Input: part model. Units: mm. Frame: model coordinates. Coordinates: 2 decimals unless noted, no trailing zeros. Write each loop counter-clockwise with the first axis right and the second up, starting at its lowest first coordinate (ties: lowest second). Pieces come first, ordered by that corner, then holes. Notation, with made-up numbers: (-3, -32.75) - (48, -32.75) arc R8 cw to (48, -21.75) - close; hole circle Ø2 at (18, 12.5). An arc over 180 degrees is marked (long way). One line per question, with ' | ' between items. Start each with the question number.
1) Section query C-C on y = 54. Return loops of the section in (x, z), and give its area (3 significant figures).
2) Section query B-B on x = -64.5. Return loops of the section in (y, z), and give its area (3 significant figures).
3) First-contact query: P1, Ø4, axis at x = -110, y = 73, coming from the +Z side; P2, Ø1.5, axis at x = 68.5, y = -59.5, coming from the -Z side; P3, Ø3, axis at x = -113.5, z = 8, coming from the +Y side. Flat tips, straight axial feed; report the tip coordinate or a pass-through.
4) Section query A-A on y = -46.5. Return loops of the section in (x, z), and give its area (3 significant figures).
5) Line query: line 1 (Z direction, x = -8.5, y = 60.5); line 2 (Y direction, x = -72, z = 8.5); line 3 (Y direction, x = -104.5, z = 6). Output: solid intervals per line, ascending.
6) Draft query along X for faces 1 (the flat face through (-2, 1, 0)), 2 (the conical face through (-117.49, -20.18, 7.24)), 3 (the conical face through (123.848, -86.434, 7.122)). Return one class per face: released by +X, released by -X, zero draft, split by the parting line, or undercut.
```python
from build123d import *

# Parameters (mm, degrees)
SKETCH_1_W      = 290
SKETCH_1_H      = 195
EXTRUDE_1_DEPTH = 5
EXTRUDE_2_DEPTH = 4
FILLET_1_R      = 5
FILLET_2_R      = 10
DRAFT_2_ANGLE   = 15
FILLET_3_R      = 2


with BuildPart() as part:
    # 草图1 → 凸台-拉伸1 (new body)
    with BuildSketch(Plane.XY):
        Rectangle(SKETCH_1_W, SKETCH_1_H)
    extrude(amount=EXTRUDE_1_DEPTH)

    # 草图2 → 凸台-拉伸2 (add)
    with BuildSketch(Plane.XY.offset(5)):
        Polygon((-75, -17.5), (-120, -17.5), (-120, -87.5), (125, -87.5), (125, -62.5), (-75, -62.5), align=None)
    extrude(amount=EXTRUDE_2_DEPTH)

    # 圆角1
    fillet_1_edges = [part.edges().sort_by_distance(p)[0] for p in [
        (-75, -62.5, 7),
        (-120, -87.5, 7),
        (125, -87.5, 7),
        (125, -62.5, 7),
    ]]
    fillet(fillet_1_edges, radius=FILLET_1_R)

    # 圆角2
    fillet_2_edges = [part.edges().sort_by_distance(p)[0] for p in [
        (-75, -17.5, 7),
        (-120, -17.5, 7),
    ]]
    fillet(fillet_2_edges, radius=FILLET_2_R)

    # 拔模2
    draft_2_faces = [part.faces().sort_by_distance(p)[0] for p in [
        (-73.535533906, -61.035533906, 7),
        (123.535533906, -63.964466094, 7),
        (123.535533906, -86.035533906, 7),
        (125, -75, 7),
        (25, -62.5, 7),
        (-75, -42.5, 7),
        (-77.928932188, -20.428932188, 7),
        (-97.5, -17.5, 7),
        (-117.071067812, -20.428932188, 7),
        (-120, -55, 7),
        (-118.535533906, -86.035533906, 7),
        (2.5, -87.5, 7),
    ]]
    draft(draft_2_faces, Plane.XY.offset(9), DRAFT_2_ANGLE)

    # 圆角3
    fillet_3_edges = [part.edges().sort_by_distance(p)[0] for p in [
        (25, -61.42820323, 5),
        (25, -62.5, 9),
        (126.07179677, -75, 5),
        (125, -75, 9),
        (-75, -42.5, 9),
        (2.5, -87.5, 9),
        (-118.535533906, -86.035533906, 9),
        (123.535533906, -86.035533906, 9),
        (123.535533906, -63.964466094, 9),
        (-73.92820323, -42.5, 5),
        (2.5, -88.57179677, 5),
        (-72.777659142, -60.277659142, 5),
        (124.29340867, -63.20659133, 5),
        (-73.535533906, -61.035533906, 9),
        (124.29340867, -86.79340867, 5),
        (-119.29340867, -86.79340867, 5),
        (-97.5, -16.42820323, 5),
        (-97.5, -17.5, 9),
        (-120, -55, 9),
        (-117.071067812, -20.428932188, 9),
        (-77.928932188, -20.428932188, 9),
        (-121.07179677, -55, 5),
        (-77.171057424, -19.671057424, 5),
        (-117.828942576, -19.671057424, 5),
    ]]
    fillet(fillet_3_edges, radius=FILLET_3_R)


solid = part.part
```
Answer key:
1) outline: (-145, 0) - (145, 0) - (145, 5) - (-145, 5) - close | area: 1,450 mm²
2) outline: (-97.5, 0) - (97.5, 0) - (97.5, 5) - (-59.89, 5) arc R2 cw to (-61.83, 6.48) - (-62.1, 7.52) arc R2 ccw to (-64.03, 9) - (-85.97, 9) arc R2 ccw to (-87.9, 7.52) - (-88.17, 6.48) arc R2 cw to (-90.11, 5) - (-97.5, 5) - close | area: 1,080 mm²
3) P1: z = 5 | P2: z = 0 | P3: y = -17.23
4) outline: (-145, 0) - (145, 0) - (145, 5) - (-72.39, 5) arc R2 cw to (-74.33, 6.48) - (-74.6, 7.52) arc R2 ccw to (-76.53, 9) - (-118.47, 9) arc R2 ccw to (-120.4, 7.52) - (-120.67, 6.48) arc R2 cw to (-122.61, 5) - (-145, 5) - close | area: 1,630 mm²
5) line 1: 0 to 5 | line 2: -87.29 to -62.31 | line 3: -88.37 to -16.63
6) face 1: zero draft | face 2: released by -X | face 3: released by +X
